```python
from build123d import *

# Parameters (mm, degrees)
BOSS_EXTRUDE1_DEPTH = 2.5
SKETCH2_W           = 0.5
SKETCH2_H           = 0.5
BOSS_EXTRUDE3_DEPTH = 5.5
SKETCH2_3_W         = 0.5
SKETCH2_3_H         = 0.5


with BuildPart() as part:
    # Sketch1 → Boss-Extrude1 (new body)
    with BuildSketch(Plane(origin=(0, 0, 0), x_dir=(1, 0, 0), z_dir=(0, 1, 0))):
        Polygon((-1.25, 0.75), (-0.75, 1.25), (0.75, 1.25), (1.25, 0.75), (1.75, 1.25), (3.25, 1.25), (3.75, 0.75), (4.25, 1.25), (5.75, 1.25), (6.25, 0.75), (6.75, 1.25), (8.25, 1.25), (8.75, 0.75), (9.25, 1.25), (10.75, 1.25), (11.25, 0.75), (11.75, 1.25), (13.25, 1.25), (13.75, 0.75), (14.25, 1.25), (15.75, 1.25), (16.25, 0.75), (16.75, 1.25), (18.25, 1.25), (18.75, 0.75), (18.75, -0.75), (18.25, -1.25), (16.75, -1.25), (16.25, -0.75), (15.75, -1.25), (14.25, -1.25), (13.75, -0.75), (13.25, -1.25), (11.75, -1.25), (11.25, -0.75), (10.75, -1.25), (9.25, -1.25), (8.75, -0.75), (8.25, -1.25), (6.75, -1.25), (6.25, -0.75), (5.75, -1.25), (4.25, -1.25), (3.75, -0.75), (3.25, -1.25), (1.75, -1.25), (1.25, -0.75), (0.75, -1.25), (-0.75, -1.25), (-1.25, -0.75), align=None)
    extrude(amount=BOSS_EXTRUDE1_DEPTH)

    # Sketch2 → Boss-Extrude3 (add)
    with BuildSketch(Plane(origin=(0, 2.5, 0), x_dir=(1, 0, 0), z_dir=(0, 1, 0))):
        with Locations((2.5, 0)):
            Rectangle(SKETCH2_W, SKETCH2_H)
        Rectangle(SKETCH2_W, SKETCH2_H)
        with Locations((5, 0)):
            Rectangle(SKETCH2_W, SKETCH2_H)
        with Locations((7.5, 0)):
            Rectangle(SKETCH2_W, SKETCH2_H)
        with Locations((10, 0)):
            Rectangle(SKETCH2_W, SKETCH2_H)
        with Locations((12.5, 0)):
            Rectangle(SKETCH2_W, SKETCH2_H)
        with Locations((15, 0)):
            Rectangle(SKETCH2_W, SKETCH2_H)
        with Locations((17.5, 0)):
            Rectangle(SKETCH2_W, SKETCH2_H)
    extrude(amount=-BOSS_EXTRUDE3_DEPTH)

    # Sweep1: sweep along a path in Sketch3
    with BuildLine(Plane(origin=(0, 0, 0), x_dir=(0, 0, -1), z_dir=(1, 0, 0))) as sweep1_path:
        Line((0, 2.5), (0, 3.5))
        ThreePointArc((0, 3.5), (-0.146446609, 3.853553391), (-0.5, 4))
        Line((-0.5, 4), (-8, 4))
    # Sketch2<3> → Sweep1 (sweep)
    with BuildSketch(Plane(origin=(0, 2.5, 0), x_dir=(1, 0, 0), z_dir=(0, 1, 0))):
        with Locations((2.5, 0)):
            Rectangle(SKETCH2_3_W, SKETCH2_3_H)
        Rectangle(SKETCH2_3_W, SKETCH2_3_H)
        with Locations((5, 0)):
            Rectangle(SKETCH2_3_W, SKETCH2_3_H)
        with Locations((7.5, 0)):
            Rectangle(SKETCH2_3_W, SKETCH2_3_H)
        with Locations((10, 0)):
            Rectangle(SKETCH2_3_W, SKETCH2_3_H)
        with Locations((12.5, 0)):
            Rectangle(SKETCH2_3_W, SKETCH2_3_H)
        with Locations((15, 0)):
            Rectangle(SKETCH2_3_W, SKETCH2_3_H)
        with Locations((17.5, 0)):
            Rectangle(SKETCH2_3_W, SKETCH2_3_H)
    sweep(path=sweep1_path.line)


solid = part.part
```
For this review, take the finished solid that the model builds, in its own axes (mm). A direction names the side the tool comes from. Coordinates: 2 decimals unless noted, no trailing zeros. Loops run counter-clockwise (first coordinate to the right, second up) from the corner with the lowest first, then second, coordinate; pieces in that order, holes last.
1. Add section C-C, the plane x = 5. Give the boundary of the cut face in (y, z).
2. Add section A-A, the plane y = -1.5. Count the separate pieces of the cut face and the enclosed holes in it, then the cut area to 3 significant figures.
3. Insertion check: P1, Ø0.6, axis at y = -1.5, z = 0, coming from the +X side; P2, Ø1.6, axis at x = -0.5, y = 2, coming from the +Z side; P3, Ø0.6, axis at y = -2, z = 0, coming from the -X side. Each pin has a flat end and moves straight along its axis. Give the tip position at first contact, or say it passes through.
4. For faces 1 (the flat face through (-0.25, 4, 3)), 2 (the flat face through (4.75, 4, 3)), 3 (the flat face through (10, 1, 1.25)), list the 3-axis set-ups (+Z, -Z, +X, -X, +Y, -Y) from which the entire face can be reached by the end or side of a thin tool; tool diameter is ignored.
5. Mouldability with a two-part tool opening along X and no side actions: class faces 4 (the flat face through (9.75, 4, 3)), 5 (the flat face through (18, 1, 1.25)), 6 (the flat face through (18.75, 1, 0)) as +X half, -X half, draft (parallel to the pull), parting line (faces both ways), or undercut.
6. For line 1 (Y direction, x = 7.5, z = 4.75); line 2 (Y direction, x = 14, z = 0.25), list the stretches that pass through material, from the lowest coordinate up.
Result:
1. outline: (-3, -0.25) - (0, -0.25) - (0, -1.25) - (2.5, -1.25) - (2.5, -0.25) - (3.5, -0.25) arc R0.75 ccw to (4.25, 0.5) - (4.25, 8) - (3.75, 8) - (3.75, 0.5) arc R0.25 cw to (3.5, 0.25) - (2.5, 0.25) - (2.5, 1.25) - (0, 1.25) - (0, 0.25) - (-3, 0.25) - close
2. separate pieces: 8
2. enclosed holes: 0
2. area: 2.00 mm2
3. P1: stops at x = 17.75
3. P2: stops at z = 1.25
3. P3: stops at x = -0.25
4. face 1: +Z, -Z, -X, +Y
4. face 2: +Z, -Z, +Y
4. face 3: +Z, +X, -X, -Y
5. face 4: undercut
5. face 5: draft
5. face 6: +X half
6. line 1: y = 3.75 to 4.25
6. line 2: y = 0 to 2.5
